```python
from build123d import *

# Parameters (mm, degrees)
SKETCH_1_R           = 34.75
SKETCH_1_R_2         = 26
EXTRUDE_1_DEPTH      = 26
EXTRUDE_2_DEPTH      = 3
EXTRUDE_2_DEPTH_BACK = 3
SKETCH_3_R           = 6
EXTRUDE_3_DEPTH      = 20
CUT_EXTRUDE_1_DEPTH  = 20


with BuildPart() as part:
    # 草图1 → 凸台-拉伸1 (new body)
    with BuildSketch(Plane(origin=(0, 0, 0), x_dir=(0, 0, -1), z_dir=(1, 0, 0))):
        with Locations(Location((0, 0, 0), (0, 0, 180))):
            Circle(SKETCH_1_R)
        with Locations(Location((0, 0, 0), (0, 0, 180))):
            Circle(SKETCH_1_R_2, mode=Mode.SUBTRACT)
    extrude(amount=EXTRUDE_1_DEPTH)

    # 草图2 → 凸台-拉伸2 (add, two sides: drawn at the far end of the back side and taken through both)
    with BuildSketch(Plane(origin=(5, 0, 0), x_dir=(0, 0, -1), z_dir=(1, 0, 0)).offset(-EXTRUDE_2_DEPTH_BACK)):
        with BuildLine():
            Line((-2.428148007, 2.428148007), (-6.441571828, 25.189405558))
            ThreePointArc((-6.441571828, 25.189405558), (0, 26), (6.441571828, 25.189405558))
            Line((6.441571828, 25.189405558), (2.428148007, 2.428148007))
            Line((2.428148007, 2.428148007), (25.189405558, 6.441571828))
            ThreePointArc((25.189405558, 6.441571828), (26, 0), (25.189405558, -6.441571828))
            Line((25.189405558, -6.441571828), (2.428148007, -2.428148007))
            Line((2.428148007, -2.428148007), (6.441571828, -25.189405558))
            ThreePointArc((6.441571828, -25.189405558), (0, -26), (-6.441571828, -25.189405558))
            Line((-6.441571828, -25.189405558), (-2.428148007, -2.428148007))
            Line((-2.428148007, -2.428148007), (-25.189405558, -6.441571828))
            ThreePointArc((-25.189405558, -6.441571828), (-26, 0), (-25.189405558, 6.441571828))
            Line((-25.189405558, 6.441571828), (-2.428148007, 2.428148007))
        make_face()
    extrude(amount=EXTRUDE_2_DEPTH + EXTRUDE_2_DEPTH_BACK)

    # 草图3 → 凸台-拉伸3 (add)
    with BuildSketch(Plane(origin=(8, 0, 0), x_dir=(0, 0, -1), z_dir=(1, 0, 0))):
        with Locations(Location((0, 0, 0), (0, 0, 150.836240305))):
            Circle(SKETCH_3_R)
    extrude(amount=EXTRUDE_3_DEPTH)

    # 草图4 → 切除-拉伸1 (cut)
    with BuildSketch(Plane(origin=(28, 0, 0), x_dir=(0, 0, -1), z_dir=(1, 0, 0))):
        with BuildLine():
            Line((-1.322875656, 1.5), (1.322875656, 1.5))
            ThreePointArc((1.322875656, 1.5), (0, -2), (-1.322875656, 1.5))
        make_face()
    extrude(amount=-CUT_EXTRUDE_1_DEPTH, mode=Mode.SUBTRACT)


solid = part.part
```
Here's how the part is built. I have some questions about the finished solid (model axes, mm). A direction names the side the tool comes from. Coordinates: 2 decimals unless noted, no trailing zeros. Loops run counter-clockwise (first coordinate to the right, second up) from the corner with the lowest first, then second, coordinate; pieces in that order, holes last. Notation, with made-up numbers: (-4, 31.25) -> (23, 31.25) arc R10 cw to (23, 44.25) -> close; hole circle Ø6 at (-22.75, -25.5). An arc over 180 degrees is marked (long way). Return JSON: item names as keys, results as strings.
1) I need wall thicknesses on line 1 (Y direction, x = 10.25, z = 0); line 2 (Z direction, x = 3, y = 20); line 3 (Z direction, x = 9.75, y = -5.5). Which ranges of each line are inside material? Lowest first, please. Write a range as from..to.
Results below:
{"line 1": "-34.75..-26, -6..-2, 1.5..6, 26..34.75", "line 2": "-28.42..-16.61, -5.53..5.53, 16.61..28.42", "line 3": "-34.31..-25.41, -2.4..2.4, 25.41..34.31"}
2) If we section it at D-D, the plane z = 0: Write out the boundary of the cut face in (x, y).
Results below:
{"outline": "(0, -34.75) -> (26, -34.75) -> (26, -26) -> (8, -26) -> (8, -6) -> (28, -6) -> (28, -2) -> (8, -2) -> (8, 1.5) -> (28, 1.5) -> (28, 6) -> (8, 6) -> (8, 26) -> (26, 26) -> (26, 34.75) -> (0, 34.75) -> (0, 26) -> (2, 26) -> (2, -26) -> (0, -26) -> close"}
3) If we section it at A-A, the plane z = 13: Write out the boundary of the cut face in (x, y).
Results below:
{"outline": "(0, -32.23) -> (26, -32.23) -> (26, -22.52) -> (0, -22.52) -> close; (0, 22.52) -> (26, 22.52) -> (26, 32.23) -> (0, 32.23) -> close; (2, -4.29) -> (8, -4.29) -> (8, 4.29) -> (2, 4.29) -> close"}
4) Will these pins go through, and if not, where does the flat tip stop? pin 1 (3 mm diameter, centred on y = -26, z = 4, fed in from -X); pin 2 (5 mm diameter, centred on x = 7.5, y = -3.5, fed in from +Z); pin 3 (3 mm diameter, centred on y = 0, z = 0, fed in from -X); pin 4 (3 mm diameter, centred on y = -26.5, z = 19.5, fed in from +X).
Results below:
{"pin 1": "x = 0", "pin 2": "z = 34.74", "pin 3": "x = 2", "pin 4": "x = 26"}
5) Thinking about a two-plate mould opening in Z: for faces 1 (the face through (28, 2, 0)), 2 (the face through (8, 0, -18)), which applies, +Z half, -Z half, draft (parallel to the pull), parting line (faces both ways), or undercut?
Results below:
{"face 1": "draft", "face 2": "undercut"}
6) If we section it at B-B, the plane x = 3.25: Write out the boundary of the cut face in (y, z).
Results below:
{"outline": "circle Ø69.5 at (0, 0); hole (-25.19, -6.44) arc R26 ccw to (-6.44, -25.19) -> (-2.43, -2.43) -> close; hole (-25.19, 6.44) -> (-2.43, 2.43) -> (-6.44, 25.19) arc R26 ccw to start; hole (2.43, -2.43) -> (6.44, -25.19) arc R26 ccw to (25.19, -6.44) -> close; hole (2.43, 2.43) -> (25.19, 6.44) arc R26 ccw to (6.44, 25.19) -> close"}
7) For faces 3 (the face through (18, 1.5, 0)), 4 (the face through (2, 0, -2)), 5 (the face through (0, 26, 5)), which set-ups out of +Z, -Z, +X, -X, +Y, -Y let a thin tool reach every point of the face, with its end or its side?
Results below:
{"face 3": "+X", "face 4": "-X", "face 5": "+Z, -Z, -X, +Y, -Y"}
8) If we section it at C-C, the plane y = 16: Write out the boundary of the cut face in (x, z).
Results below:
{"outline": "(0, -30.85) -> (26, -30.85) -> (26, -20.49) -> (0, -20.49) -> close; (0, 20.49) -> (26, 20.49) -> (26, 30.85) -> (0, 30.85) -> close; (2, -4.82) -> (8, -4.82) -> (8, 4.82) -> (2, 4.82) -> close"}
